```python
from build123d import *

# Parameters (mm, degrees)
EXTRUDE_1_DEPTH     = 15
SKETCH_2_R          = 4
CUT_EXTRUDE_1_DEPTH = 4
SKETCH_2_3_R        = 4
CUT_EXTRUDE_2_DEPTH = 16


with BuildPart() as part:
    # Эскиз1 → Бобышка-Вытянуть1 (new body)
    with BuildSketch(Plane.XY):
        with BuildLine():
            Line((8.637636339, 2.528089888), (3.838949484, 18.923595506))
            ThreePointArc((3.838949484, 18.923595506), (0, 21.8), (-3.838949484, 18.923595506))
            Line((-3.838949484, 18.923595506), (-8.637636339, 2.528089888))
            ThreePointArc((-8.637636339, 2.528089888), (0, -9), (8.637636339, 2.528089888))
        make_face()
    extrude(amount=EXTRUDE_1_DEPTH)

    # Эскиз2 → Вырез-Вытянуть1 (cut)
    with BuildSketch(Plane(origin=(0, 0, 0), x_dir=(-1, 0, 0), z_dir=(0, 0, -1))):
        with BuildLine():
            Line((4.737753812, 4.302753632), (2.6, 17.8))
            ThreePointArc((2.6, 17.8), (0, 20.4), (-2.6, 17.8))
            Line((-2.6, 17.8), (-4.737753812, 4.302753632))
            ThreePointArc((-4.737753812, 4.302753632), (0, -6.4), (4.737753812, 4.302753632))
        make_face()
        Circle(SKETCH_2_R, mode=Mode.SUBTRACT)
    extrude(amount=-CUT_EXTRUDE_1_DEPTH, mode=Mode.SUBTRACT)

    # Эскиз2<3> → Вырез-Вытянуть2 (cut, through all)
    with BuildSketch(Plane(origin=(0, 0, 0), x_dir=(-1, 0, 0), z_dir=(0, 0, -1))):
        Circle(SKETCH_2_3_R)
    extrude(amount=-CUT_EXTRUDE_2_DEPTH, mode=Mode.SUBTRACT)


solid = part.part
```
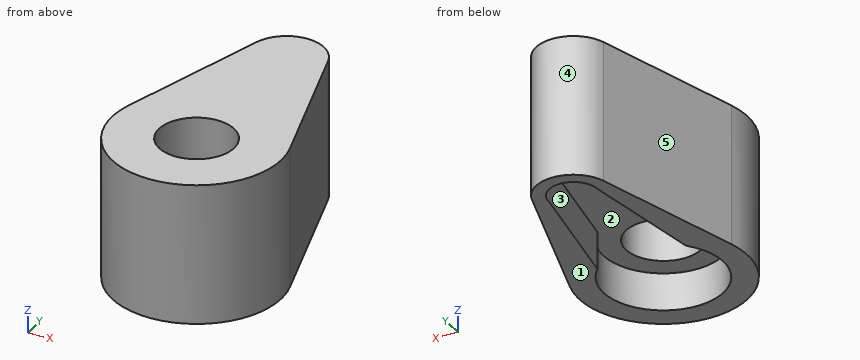
Can you work these out from the model? Positions are in its coordinate system, mm. Face numbers are marked on the shaded views. A direction names the side the tool comes from. Coordinates: 2 decimals unless noted, no trailing zeros. Loops run counter-clockwise (first coordinate to the right, second up) from the corner with the lowest first, then second, coordinate; pieces in that order, holes last. Notation, with made-up numbers: (22, -3) - (56, -3) arc R5 ccw to (56, 4) - close; hole circle Ø1 at (72.25, -6). An arc over 180 degrees is marked (long way). Answer as CSV lines item,"result". Start each with the question number.
1) Suppose I cut it at C-C (z = 1.5). Please give me the cut outline in (x, y).
2) For pin 1 (4 mm diameter, centred on y = -4, z = 8, fed in from -X); pin 2 (3 mm diameter, centred on y = -6, z = 5.5, fed in from +X); pin 3 (1.5 mm diameter, centred on x = -1, y = 11, fed in from -Z), each with a flat end and sliding along its axis, tell me the tip position at first contact or that it passes through.
3) Suppose I cut it at B-B (x = 0). Please give me the cut outline in (y, z).
4) Suppose I cut it at A-A (y = 0). Please give me the cut outline in (x, z), plus the area to 3 significant figures.
5) Thinking about a two-plate mould opening in X: for the marked faces 3, 4 and 5, which applies, pulls with the +X half, pulls with the -X half, needs draft (parallel to the pull), parting line crosses it, or undercut?
6) I need wall thicknesses on line 1 (Y direction, x = 0.25, z = 4.5); line 2 (X direction, y = 0, z = 1.45); line 3 (Z direction, x = 1, y = 9). Which ranges of each line are inside material? Lowest first, please. Write a range as from..to.
7) Which directions (+Z, -Z, +X, -X, +Y, -Y) give clear straight access to the entire face, cutting with the end or side of a thin tool? Please do the marked faces 1 and 2.
8) Suppose I cut it at D-D (y = 8). Please give me the cut outline in (x, z).
Check result:
1,outline,"(-8.64, 2.53) arc R9 ccw (long way) to (8.64, 2.53) - (3.84, 18.92) arc R4 ccw to (-3.84, 18.92) - close; hole (-4.74, 4.3) arc R6.4 ccw (long way) to (4.74, 4.3) - (2.6, 17.8) arc R2.6 ccw to (-2.6, 17.8) - close"
2,pin 1,"stops at x = -8.77"
2,pin 2,"stops at x = 7.79"
2,pin 3,"stops at z = 4"
3,outline,"(-9, 0) - (-6.4, 0) - (-6.4, 4) - (-4, 4) - (-4, 15) - (-9, 15) - close; (4, 4) - (20.4, 4) - (20.4, 0) - (21.8, 0) - (21.8, 15) - (4, 15) - close"
4,outline,"(-9, 0) - (-6.4, 0) - (-6.4, 4) - (-4, 4) - (-4, 15) - (-9, 15) - close; (4, 4) - (6.4, 4) - (6.4, 0) - (9, 0) - (9, 15) - (4, 15) - close"
4,area,"131 mm²"
5,face 3,"undercut"
5,face 4,"parting line crosses it"
5,face 5,"pulls with the -X half"
6,line 1,"y = -9..-3.99, 3.99..21.79"
6,line 2,"x = -9..-6.4, 6.4..9"
6,line 3,"z = 4..15"
7,face 1,"-Z, +X, -X, +Y, -Y"
7,face 2,"-Z"
8,outline,"(-7.04, 0) - (-4.15, 0) - (-4.15, 4) - (4.15, 4) - (4.15, 0) - (7.04, 0) - (7.04, 15) - (-7.04, 15) - close"
